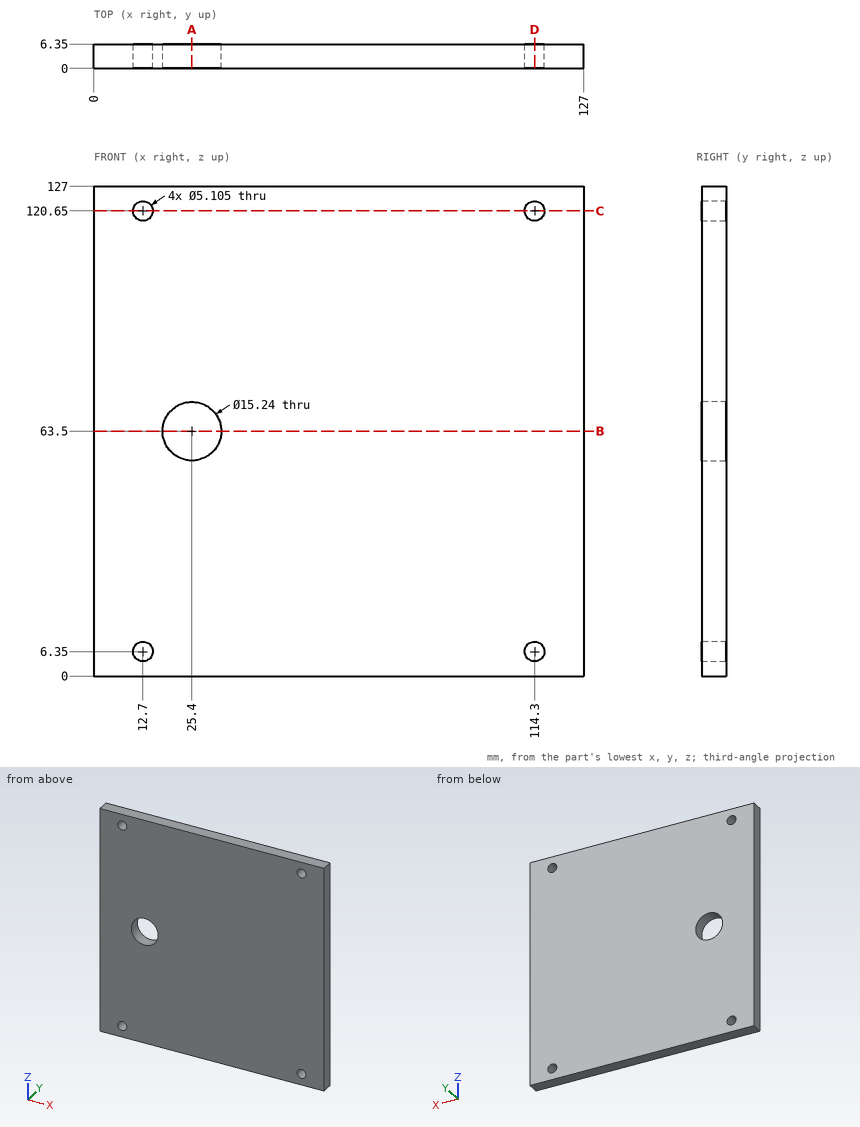
The drawing under review shows one solid part. Ordinate dimensions are in mm from its lowest x, y, z. Round coordinates to 2 decimals unless told otherwise and drop trailing zeros. Loops run counter-clockwise (first coordinate to the right, second up) from the corner with the lowest first, then second, coordinate; pieces in that order, holes last. Notation, with made-up numbers: (50, -12) - (98, -12) arc R7 cw to (98, 1) - close; hole circle Ø10 at (8.5, 1.5). An arc over 180 degrees is marked (long way). Put each result on its own line as item: value. Start each with the question number.
1. Consider section A-A on x = 25.4. State the section outline as (y, z) points.
2. For probe 1 along X at (y, z) = (5, 120.65); probe 2 along X at (y, z) = (2.75, 120), list the stretches that pass through material, from the lowest coordinate up. Write a range as [from, to].
3. Insertion check: P1, Ø6, axis at x = 14, z = 49, coming from the -Y side; P2, Ø12, axis at x = 25.4, z = 63.5, coming from the -Y side. Each pin has a flat end and moves straight along its axis. Give the tip position at first contact, or say it passes through.
4. Consider section C-C on z = 120.65. State the section outline as (x, y) points.
5. Consider section B-B on z = 63.5. State the section outline as (x, y) points.
6. Consider section D-D on x = 114.3. State the section outline as (y, z) points.
Result sheet:
1. outline: (0, 0) - (6.35, 0) - (6.35, 55.88) - (0, 55.88) - close; (0, 71.12) - (6.35, 71.12) - (6.35, 127) - (0, 127) - close
2. probe 1: [0, 10.15], [15.25, 111.75], [116.85, 127]
2. probe 2: [0, 10.23], [15.17, 111.83], [116.77, 127]
3. P1: y = 0
3. P2: through
4. outline: (0, 0) - (10.15, 0) - (10.15, 6.35) - (0, 6.35) - close; (15.25, 0) - (111.75, 0) - (111.75, 6.35) - (15.25, 6.35) - close; (116.85, 0) - (127, 0) - (127, 6.35) - (116.85, 6.35) - close
5. outline: (0, 0) - (17.78, 0) - (17.78, 6.35) - (0, 6.35) - close; (33.02, 0) - (127, 0) - (127, 6.35) - (33.02, 6.35) - close
6. outline: (0, 0) - (6.35, 0) - (6.35, 3.8) - (0, 3.8) - close; (0, 8.9) - (6.35, 8.9) - (6.35, 118.1) - (0, 118.1) - close; (0, 123.2) - (6.35, 123.2) - (6.35, 127) - (0, 127) - close
